Autodesk Inventor part; units mm, degrees
ref_plane "YZ Plane" through (0, 0, 0) normal (1, 0, 0) x (0, 1, 0)
ref_plane "XZ Plane" through (0, 0, 0) normal (0, 1, 0) x (-1, 0, 0)
ref_plane "XY Plane" through (0, 0, 0) normal (0, 0, 1) x (1, 0, 0)
sketch "Sketch1" plane through (0, 0, 0) normal (0, 1, 0) x (-1, 0, 0)
  line L0 (9.25, -9.25) -> (-9.25, -9.25)
  line L1 (-9.25, -9.25) -> (-9.25, 9.25)
  line L2 (-9.25, 9.25) -> (9.25, 9.25)
  line L3 (9.25, 9.25) -> (9.25, -9.25)
  point P0 (0, 0)
  point P1 (0, 0)
  dimension "d0" = 18.5
extrude "Extrusion1" add sketch "Sketch1" along normal blind 10
fillet "Fillet1" radius 2.5 4 edges at (9.25, 5, 9.25) (-9.25, 5, 9.25) (9.25, 5, -9.25) (-9.25, 5, -9.25)
sketch "Sketch2" plane through (0, 10, 0) normal (0, 1, 0) x (1, 0, 0)
  circle A0 centre (0, 0) radius 2.5
  dimension "d4" = 5
extrude "Extrusion2" cut sketch "Sketch2" against normal through all
sketch "Sketch3" plane through (0, 10, 0) normal (0, 1, 0) x (1, 0, 0)
  line L0 (-1.5, -2.5) -> (1.5, -2.5)
  line L1 (1.5, -2.5) -> (1.5, 2.5)
  line L2 (1.5, 2.5) -> (-1.5, 2.5)
  line L3 (-1.5, 2.5) -> (-1.5, -2.5)
  line L4 (-1.5, -2.5) -> (1.5, 2.5) construction
  line L5 (1.5, -2.5) -> (-1.5, 2.5) construction
  line L6 (-3.8508, -4.7625) -> (3.8508, -4.7625)
  line L7 (3.8508, -4.7625) -> (3.8508, 4.7625)
  line L8 (3.8508, 4.7625) -> (-3.8508, 4.7625)
  line L9 (-3.8508, 4.7625) -> (-3.8508, -4.7625)
  line L10 (-3.8508, -4.7625) -> (3.8508, 4.7625) construction
  line L11 (3.8508, -4.7625) -> (-3.8508, 4.7625) construction
  point P0 (0, 0)
  point P1 (0, 0)
  dimension "d7" = 3
extrude "Extrusion3" add sketch "Sketch3" against normal blind 7.5
properties part number "servo connector"
Input: part model. Units: mm. Frame: model coordinates. A direction names the side the tool comes from. Coordinates: 2 decimals unless noted, no trailing zeros. Loops run counter-clockwise (first coordinate to the right, second up) from the corner with the lowest first, then second, coordinate; pieces in that order, holes last. Notation, with made-up numbers: (54.5, 17.5) -> (70.5, 17.5) arc R19 cw to (70.5, 33.5) -> close; hole circle Ø3 at (61.25, 49.25). An arc over 180 degrees is marked (long way). Write item = value, one per line. Start each with the question number.
Item 1: Reachability of faces 1 (the face through (1.34, 3.96, -2.11)), 2 (the face through (-1.5, 6, 0)), 3 (the face through (-9.25, 5, 0)) from +Z, -Z, +X, -X, +Y, -Y: full face, straight path, thin tool, end or side. Return the list, or none.
Item 2: Cut plane C-C, the plane y = 6.5. Return loops of the section in (x, z), plus the area to 3 significant figures.
Item 3: Material intervals for line 1 (X direction, y = 4, z = 0); line 2 (Z direction, x = 0, y = 2); line 3 (Y direction, x = 1.75, z = 0.25), sorted ascending.
Item 4: Cut plane D-D, the plane y = 1.5. Return loops of the section in (x, z).
Item 5: Cut plane B-B, the plane z = 0. Return loops of the section in (x, y).
Item 6: Mould query, pull axis Z, two halves, no side actions, for faces 4 (the face through (2, 2.5, 0)), 5 (the face through (-2, 2.5, 0)), 6 (the face through (8.537, 5.07, -8.498)), 7 (the face through (9.25, 5, 0)). Classes: pulls with the +Z half, pulls with the -Z half, needs draft (parallel to the pull), parting line crosses it, or undercut.
Item 7: Cut plane A-A, the plane x = 0. Return loops of the section in (y, z).
Ans:
q1.face_1 = -Y
q1.face_2 = +Y, -Y
q1.face_3 = +Z, -Z, -X, +Y, -Y
q2.outline = (-9.25, -6.75) arc R2.5 ccw to (-6.75, -9.25) -> (6.75, -9.25) arc R2.5 ccw to (9.25, -6.75) -> (9.25, 6.75) arc R2.5 ccw to (6.75, 9.25) -> (-6.75, 9.25) arc R2.5 ccw to (-9.25, 6.75) -> close; hole (-1.5, -2) arc R2.5 ccw to (1.5, -2) -> (1.5, 2) arc R2.5 ccw to (-1.5, 2) -> close
q2.area = 323 mm²
q3.line_1 = -9.25 to -1.5, 1.5 to 9.25
q3.line_2 = -9.25 to -2.5, 2.5 to 9.25
q3.line_3 = 2.5 to 10
q4.outline = (-9.25, -6.75) arc R2.5 ccw to (-6.75, -9.25) -> (6.75, -9.25) arc R2.5 ccw to (9.25, -6.75) -> (9.25, 6.75) arc R2.5 ccw to (6.75, 9.25) -> (-6.75, 9.25) arc R2.5 ccw to (-9.25, 6.75) -> close; hole circle Ø5 at (0, 0)
q5.outline = (-9.25, 0) -> (-2.5, 0) -> (-2.5, 2.5) -> (-1.5, 2.5) -> (-1.5, 10) -> (-9.25, 10) -> close; (1.5, 2.5) -> (2.5, 2.5) -> (2.5, 0) -> (9.25, 0) -> (9.25, 10) -> (1.5, 10) -> close
q6.face_4 = undercut
q6.face_5 = undercut
q6.face_6 = pulls with the -Z half
q6.face_7 = needs draft
q7.outline = (0, -9.25) -> (10, -9.25) -> (10, -2.5) -> (0, -2.5) -> close; (0, 2.5) -> (10, 2.5) -> (10, 9.25) -> (0, 9.25) -> close
